Autodesk Inventor part; units mm, degrees
ref_plane "YZ Plane" through (0, 0, 0) normal (1, 0, 0) x (0, 1, 0)
ref_plane "XZ Plane" through (0, 0, 0) normal (0, 1, 0) x (-1, 0, 0)
ref_plane "XY Plane" through (0, 0, 0) normal (0, 0, 1) x (1, 0, 0)
sketch "Sketch1" plane through (0, 0, 0) normal (0, 0, 1) x (1, 0, 0)
  line L0 (-15.2972, 20.3009) -> (-2.5972, 20.3009)
  line L1 (-2.5972, 20.3009) -> (-2.5972, -5.0991)
  line L2 (-1.0722, -17.7991) -> (-15.2972, -17.7991)
  line L3 (-15.2972, -17.7991) -> (-15.2972, 20.3009)
  line L4 (-2.5972, -5.0991) -> (21.4362, -5.0991)
  line L5 (21.4362, -5.0991) -> (21.4362, -17.7991)
  line L6 (21.4362, -17.7991) -> (-1.0722, -17.7991)
  point P0 (0, 0)
  dimension "d0" = 38.1
  dimension "d1" = 12.7
  dimension "d2" = 25.4
extrude "Extrusion1" add sketch "Sketch1" along normal blind 38.1
chamfer "Chamfer1" distance 3.175 angle 45 1 edges at (-2.5972, 20.3009, 19.05)
chamfer "Chamfer2" distance 6.35 angle 45 1 edges at (21.4362, -5.0991, 19.05)
fillet "Fillet2" radius 3.175 1 edges at (-2.5972, -5.0991, 19.05)
properties part number "ChamferAngle"
The model under review builds one solid part; all positions refer to its coordinate system, in mm. A direction names the side the tool comes from. Give positions to 0.01 mm unless a question says otherwise; leave off trailing zeros. Loops run counter-clockwise (first coordinate to the right, second up) from the corner with the lowest first, then second, coordinate; pieces in that order, holes last. Notation, with made-up numbers: (-36.75, 54.5) -> (9.25, 54.5) arc R21 cw to (9.25, 81.5) -> close; hole circle Ø9 at (8, -29). An arc over 180 degrees is marked (long way). Use CSV: the item, a comma, the result in double quotes.
1. Consider section C-C, the plane y = 7.5. Write out the cut boundary in (x, z).
Result:
outline,"(-15.3, 0) -> (-2.6, 0) -> (-2.6, 38.1) -> (-15.3, 38.1) -> close"
2. Machinability: for faces 1 (the face through (8, -5.099, 19)), 2 (the face through (21.436, -15, 19)), which of the approach directions +Z, -Z, +X, -X, +Y, -Y give a long, thin tool a straight path to every point of the face, cutting with its end or side? Answer none if there is none.
Result:
face 1,"+Z, -Z, +X, +Y"
face 2,"+Z, -Z, +X, +Y, -Y"
3. For P1, Ø6, axis at y = 1.5, z = 8.5, coming from the +X side; P2, Ø16, axis at x = 6.5, z = 17.5, coming from the +Y side; P3, Ø2, axis at x = 3, z = 11.5, coming from the +Y side, all flat-tipped, find the tip position at first contact; note any pin that passes through.
Result:
P1,"stops at x = -2.6"
P2,"stops at y = -4.32"
P3,"stops at y = -5.1"
4. Consider section B-B, the plane x = 7. Write out the cut boundary in (y, z), then the cut area to 3 significant figures.
Result:
outline,"(-17.8, 0) -> (-5.1, 0) -> (-5.1, 38.1) -> (-17.8, 38.1) -> close"
area,"484 mm²"
5. Consider section A-A, the plane z = 18.5. Write out the cut boundary in (x, y) (3 decimals), then the cut area to 3 significant figures.
Result:
outline,"(-15.297, -17.799) -> (21.436, -17.799) -> (21.436, -11.449) -> (15.086, -5.099) -> (0.578, -5.099) arc R3.175 cw to (-2.597, -1.924) -> (-2.597, 17.126) -> (-5.772, 20.301) -> (-15.297, 20.301) -> close"
area,"766 mm²"
6. To check wall thickness, follow probe 1 along X at (y, z) = (16, 29); probe 2 along Y at (x, z) = (12, 29); probe 3 along Y at (x, z) = (17, 19). State the ranges of each line that lie inside material, in increasing order. Write a range as from..to.
Result:
probe 1,"x = -15.3..-2.6"
probe 2,"y = -17.8..-5.1"
probe 3,"y = -17.8..-7.01"
